Geometry: final body of the model. Coordinates: model frame, mm. Round coordinates to 2 decimals unless told otherwise and drop trailing zeros. Write each loop counter-clockwise with the first axis right and the second up, starting at its lowest first coordinate (ties: lowest second). Pieces come first, ordered by that corner, then holes. Notation, with made-up numbers: M -34.5,15.5 L -6.5,15.5 A21 ccw -6.5,38.5 Z; hole C 66,89.5 d9. An arc over 180 degrees is marked long. Put each result on its own line as item: value. Start each with the question number.
```python
from build123d import *

# Parameters (mm, degrees)
F2_DEPTH = 12.7
F3_SIZE  = 5.2832
F0_R     = 2.286


with BuildPart() as f2:
    # F1 (on Top) → F2 (new body)
    with BuildSketch(Plane.XY):
        Polygon((10.633536, 11.875212), (0, 26.371382), (0.358835, -20.400941), (10.128893, -13.75857), align=None)
        Polygon((0.358835, -20.400941), (0, 26.371382), (-10.409869, 11.713768), (-9.511987, -13.909254), align=None)
    extrude(amount=F2_DEPTH)

    # F3
    f3_edges = [f2.edges().sort_by_distance(p)[0] for p in [
        (-9.960928, -1.097743, 12.7),
        (-4.576576, -17.155098, 12.7),
        (5.243864, -17.079756, 12.7),
        (10.381214, -0.941679, 12.7),
        (5.316768, 19.123297, 12.7),
        (-5.204935, 19.042575, 12.7),
    ]]
    chamfer(f3_edges, length=F3_SIZE)

    # F0
    f0_edges = [f2.edges().sort_by_distance(p)[0] for p in [
        (0.358835, -20.400941, 3.7084),
    ]]
    fillet(f0_edges, radius=F0_R)


solid = f2.part
```
1) Ray query, probe 1 along Y at (x, z) = (-1, 4); probe 2 along Y at (x, z) = (4, 2.25); probe 3 along X at (y, z) = (-12, 8.75). Return the intervals inside material, ascending.
2) Section C-C, the plane x = 8.75. Output: boundary loops of the cut face in (y, z).
3) Section D-D, the plane z = 8.5. Output: boundary loops of the cut face in (x, y), and give its area (3 significant figures).
4) Section B-B, the plane y = 11. Output: boundary loops of the cut face in (x, z), and give its area (3 significant figures).
5) Section A-A, the plane z = 6.5. Output: boundary loops of the cut face in (x, y), and give its area (3 significant figures).
6) First-contact query: pin 1 (3 mm diameter, centred on x = 2.5, z = 11, fed in from -Y); pin 2 (2 mm diameter, centred on x = -4, z = 9.5, fed in from -Y); pin 3 (4 mm diameter, centred on y = -0.5, z = 5, fed in from +X). Flat tips, straight axial feed; report the tip coordinate or a pass-through.
Solved:
1. probe 1: y = -19.51 to 24.96
1. probe 2: y = -17.93 to 20.92
1. probe 3: x = -8.24 to 8.83
2. outline: M -14.7,0 L 14.44,0 L 14.44,7.42 L 11.28,9.29 L -13.01,8.81 L -14.7,7.42 Z
3. outline: M -9.31,11.39 L -8.45,-13.31 L 0.35,-19.1 L 9.06,-13.18 L 9.54,11.53 L 0.01,24.52 Z
3. area: 624 mm2
4. outline: M -10.38,0 L 10.62,0 L 10.62,7.42 L 7.87,10.16 L 4.72,12.7 L -4.44,12.7 L -8.03,9.77 L -10.38,7.42 Z
4. area: 237 mm2
5. outline: M -10.41,11.71 L -9.51,-13.91 L -0.92,-19.56 A2.29 ccw 1.62,-19.54 L 10.13,-13.76 L 10.63,11.88 L 0,26.37 Z
5. area: 739 mm2
6. pin 1: stops at y = -16.69
6. pin 2: stops at y = -16.41
6. pin 3: stops at x = 10.43
